Autodesk Inventor part; units mm, degrees
ref_plane "XZ Plane" through (0, 0, 0) normal (0, 1, 0) x (-1, 0, 0)
ref_plane "XY Plane" through (0, 0, 0) normal (0, 0, 1) x (1, 0, 0)
sketch "Szkic1" plane through (0, 0, 0) normal (0, 1, 0) x (-1, 0, 0)
  circle A0 centre (0, 0) radius 4.25
  dimension "d0" = 8.5
extrude "Wyciągnięcie proste1" add sketch "Szkic1" along normal mid plane 5
sketch "Szkic2" plane through (0, 2.5, 0) normal (0, 1, 0) x (1, 0, 0)
  circle A0 centre (0, 0) radius 2.55
  dimension "d3" = 5.1
extrude "Wyciągnięcie proste2" add sketch "Szkic2" along normal blind 60
ref_plane "Płaszczyzna konstrukcyjna1" through (-2.65, 0, 0) normal (1, 0, 0) x (0, 1, 0)
sketch "Szkic3" plane through (-2.65, 0, 0) normal (1, 0, 0) x (0, 1, 0)
  point P0 (0, 0)
sketch "Szkic4" plane through (-2.65, 0, 0) normal (1, 0, 0) x (0, 1, 0)
  circle A0 centre (52.5, 0) radius 1.55
  line L0 (62.5, -2.55) -> (62.5, 2.55)
  point P0 (0, 0)
  dimension "d8" = 3.1
  dimension "d9" = 10
extrude "Wyciągnięcie proste3" cut sketch "Szkic4" along normal blind 50
properties part number "sworzen"
Work out the finished part from the listing and answer in its coordinate system (mm). A direction names the side the tool comes from. Round coordinates to 2 decimals unless told otherwise and drop trailing zeros. Loops run counter-clockwise (first coordinate to the right, second up) from the corner with the lowest first, then second, coordinate; pieces in that order, holes last. Notation, with made-up numbers: (59.5, 39.25) - (98.5, 39.25) arc R29 ccw to (98.5, 78.25) - close; hole circle Ø7 at (16, 33). An arc over 180 degrees is marked (long way). Use one line per item in the form item = value. Start each with the question number.
(1) Find section B-B on x = 0. Determine the outline of the cut face in (y, z), and give its area (3 significant figures).
(2) Consider line 1 (Y direction, x = 0.05, z = 0); line 2 (Y direction, x = -0.5, z = -3); line 3 (Z direction, x = 1.1, y = 52.5). Determine where each line is inside the solid, lowest interval first.
(3) Find section C-C on y = 21.5. Determine the outline of the cut face in (x, z), and give its area (3 significant figures).
(4) Determine the mould class of faces 1 (the face through (-2.548, 32.08, 0.112)), 2 (the face through (-0.04, 50.95, -0.07)), 3 (the face through (0, -2.5, 0)) for opening direction Y: +Y half, -Y half, draft (parallel to the pull), parting line (faces both ways), or undercut.
(5) Which of the six approach directions +Z, -Z, +X, -X, +Y, -Y give full straight-line access (tool end or side, diameter ignored) to faces 4 (the face through (-2, 2.5, -2)), 5 (the face through (-2.285, -0.035, -3.584))?
(6) Find section A-A on z = 0. Determine the outline of the cut face in (x, y).
(7) Find section D-D on y = 52.5. Determine the outline of the cut face in (x, z).
(8) Flat-ended cylindrical pins translate along their axes: P1, Ø5, axis at x = -3, y = 34, coming from the +Z side; P2, Ø2.5, axis at y = 52.5, z = 0, coming from the -X side. Find the tip coordinate at first contact, or state that the pin passes through.
Answer list:
q1.outline = (-2.5, -4.25) - (2.5, -4.25) - (2.5, -2.55) - (62.5, -2.55) - (62.5, 2.55) - (2.5, 2.55) - (2.5, 4.25) - (-2.5, 4.25) - close; hole circle Ø3.1 at (52.5, 0)
q1.area = 341 mm^2
q2.line_1 = -2.5 to 50.95, 54.05 to 62.5
q2.line_2 = -2.5 to 2.5
q2.line_3 = -2.3 to -1.55, 1.55 to 2.3
q3.outline = circle Ø5.1 at (0, 0)
q3.area = 20.4 mm^2
q4.face_1 = draft
q4.face_2 = undercut
q4.face_3 = -Y half
q5.face_4 = +Y
q5.face_5 = +Y, -Y
q6.outline = (-4.25, -2.5) - (4.25, -2.5) - (4.25, 2.5) - (2.55, 2.5) - (2.55, 50.95) - (-2.55, 50.95) - (-2.55, 2.5) - (-4.25, 2.5) - close; (-2.55, 54.05) - (2.55, 54.05) - (2.55, 62.5) - (-2.55, 62.5) - close
q7.outline = (-2.02, -1.55) arc R2.55 ccw to (2.02, -1.55) - close; (-2.02, 1.55) - (2.02, 1.55) arc R2.55 ccw to start
q8.P1 = 2.5
q8.P2 = through
